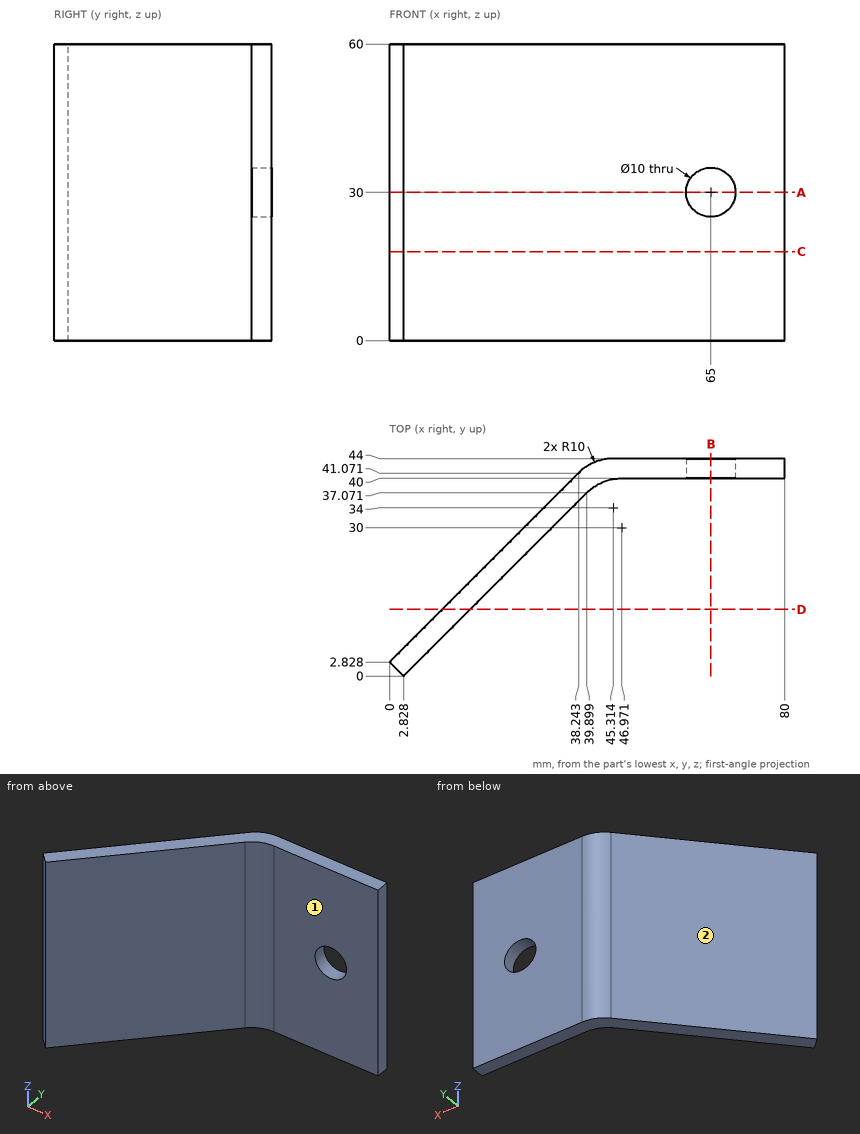
Verification items for this drawing (mm, ordinates from the low corner). A direction names the side the tool comes from. Coordinates: 2 decimals unless noted, no trailing zeros. Order: outer loops, then holes, each group sorted by start corner. A loop starts at its lowest first (then second) coordinate and runs counter-clockwise, first axis right, second up. Notation, with made-up numbers: (39.5, 46) - (69.5, 46) arc R33 ccw to (69.5, 76) - close; hole circle Ø7 at (-38.5, 65.25). An arc over 180 degrees is marked (long way). Answer in a Markdown table with one row per item. Add a question column.
1. Section check B-B (x = 65). Enter the section's corners in (y, z), plus the area to 3 significant figures.
2. Section check A-A (z = 30). Enter the section's corners in (x, y).
3. Section check C-C (z = 18). Enter the section's corners in (x, y).
4. Gauge pin test, flat ends, axial feed: pin 1 Ø10 at (x, z) = (68, 20.5) entering from -Y; pin 2 Ø12 at (y, z) = (15.5, 52.5) entering from +X; pin 3 Ø8 at (y, z) = (12, 47.5) entering from +X; pin 4 Ø8 at (x, y) = (71, 33.5) entering from +Z. Record the tip position at first contact, or that the pin passes through.
5. Material ranges on L1, parallel to Z at x = 65, y = 42; L2, parallel to Y at x = 72.5, z = 23; L3, parallel to X at y = 30, z = 51.5, recorded low to high. Write a range as [from, to].
6. Section check D-D (y = 13.5). Enter the section's corners in (x, z).
7. Access from +Z, -Z, +X, -X, +Y, -Y to the whole of each face (thin tool, end or side, straight path). Record for the marked faces 1 and 2.
Data:
| question | item | result |
|---|---|---|
| 1 | outline | (40, 0) - (44, 0) - (44, 25) - (40, 25) - close; (40, 35) - (44, 35) - (44, 60) - (40, 60) - close |
| 1 | area | 200 mm² |
| 2 | outline | (0, 2.83) - (2.83, 0) - (39.9, 37.07) arc R10 cw to (46.97, 40) - (60, 40) - (60, 44) - (45.31, 44) arc R10 ccw to (38.24, 41.07) - close; (70, 40) - (80, 40) - (80, 44) - (70, 44) - close |
| 3 | outline | (0, 2.83) - (2.83, 0) - (39.9, 37.07) arc R10 cw to (46.97, 40) - (80, 40) - (80, 44) - (45.31, 44) arc R10 ccw to (38.24, 41.07) - close |
| 4 | pin 1 | stops at y = 40 |
| 4 | pin 2 | stops at x = 24.33 |
| 4 | pin 3 | stops at x = 18.83 |
| 4 | pin 4 | passes through |
| 5 | L1 | z = [0, 25], [35, 60] |
| 5 | L2 | y = [40, 44] |
| 5 | L3 | x = [27.17, 32.83] |
| 6 | outline | (10.67, 0) - (16.33, 0) - (16.33, 60) - (10.67, 60) - close |
| 7 | face 1 | +Z, -Z, +X, -Y |
| 7 | face 2 | +Z, -Z, -X, +Y |
